from build123d import *

# Parameters (mm, degrees)
F0_R     = 30
F1_DEPTH = 1
F2_R     = 22.5
F3_DEPTH = 24
F5_R     = 20
F6_DEPTH = 25.001


# Not quite as in the source:
# - the program builds the solid bodies; features that only make, move or delete a surface that nothing else refers to are left out


with BuildPart() as f1:
    # F0 (on Front) → F1 (new body)
    with BuildSketch(Plane.XZ):
        Circle(F0_R)
    extrude(amount=F1_DEPTH)

    # F2 (on face) → F3 (join)
    with BuildSketch(Plane.XZ.offset(1)):
        Circle(F2_R)
    extrude(amount=F3_DEPTH)

    # F5 (on face) → F6 (cut, through all)
    with BuildSketch(Plane.XZ.offset(25)):
        Circle(F5_R)
    extrude(amount=-F6_DEPTH, mode=Mode.SUBTRACT)


solid = f1.part
Work out the finished part from the listing and answer in its coordinate system (mm). A direction names the side the tool comes from. Coordinates: 2 decimals unless noted, no trailing zeros. Write each loop counter-clockwise with the first axis right and the second up, starting at its lowest first coordinate (ties: lowest second). Pieces come first, ordered by that corner, then holes. Notation, with made-up numbers: M 35,34 L 57,34 A19 ccw 57,70 Z; hole C 47.25,81.5 d10. An arc over 180 degrees is marked long. Write item = value, one per line.
1. Straight lines are drawn through the part: line 1 (Z direction, x = 0, y = -15.75); line 2 (Z direction, x = 9, y = -17.25); line 3 (Y direction, x = 24.5, z = 1). For each, find the intervals that lie inside material, in ascending order. Write a range as from..to.
Solution:
line_1 = -22.5..-20, 20..22.5
line_2 = -20.62..-17.86, 17.86..20.62
line_3 = -1..0
2. The part is cut by section A-A (z = 0). Determine the outline of the cut face in (x, y), then the cut area to 3 significant figures.
Solution:
outline = M -30,-1 L -22.5,-1 L -22.5,-25 L -20,-25 L -20,0 L -30,0 Z; M 20,-25 L 22.5,-25 L 22.5,-1 L 30,-1 L 30,0 L 20,0 Z
area = 140 mm2
3. The part is cut by section D-D (x = -21.5). Determine the outline of the cut face in (y, z), then the cut area to 3 significant figures.
Solution:
outline = M -25,-6.63 L -1,-6.63 L -1,-20.92 L 0,-20.92 L 0,20.92 L -1,20.92 L -1,6.63 L -25,6.63 Z
area = 360 mm2
4. For faces 4 (the face through (6, 0, -20)), 5 (the face through (10.382, -12.832, -19.961)), determine the directions among +Z, -Z, +X, -X, +Y, -Y from which every point of the face is accessible in a straight line to the end or side of a thin tool.
Solution:
face_4 = +Z, -Z, +X, -X, +Y
face_5 = -Y
5. The part is cut by section B-B (x = 0). Determine the outline of the cut face in (y, z), then the cut area to 3 significant figures.
Solution:
outline = M -25,-22.5 L -1,-22.5 L -1,-30 L 0,-30 L 0,-20 L -25,-20 Z; M -25,20 L 0,20 L 0,30 L -1,30 L -1,22.5 L -25,22.5 Z
area = 140 mm2
6. The part is cut by section C-C (y = -20.75). Determine the outline of the cut face in (x, z), then the cut area to 3 significant figures.
Solution:
outline = C 0,0 d45; hole C 0,0 d40
area = 334 mm2
7. Determine the mould class of faces 1 (the face through (-4.336, -12.675, -19.524)), 2 (the face through (4.3, -1, 22.4)), 3 (the face through (-29.97, -0.49, 1.32)) for opening direction X: released by +X, released by -X, zero draft, split by the parting line, or undercut.
Solution:
face_1 = undercut
face_2 = zero draft
face_3 = split by the parting line
8. Flat-ended cylindrical pins translate along their axes: pin 1 (1 mm diameter, centred on x = 6.5, y = -22.5, fed in from +Z); pin 2 (8 mm diameter, centred on y = -10, z = -0.5, fed in from +X); pin 3 (1.5 mm diameter, centred on x = -20, y = -8.5, fed in from -Z); pin 4 (24 mm diameter, centred on x = 0, z = 0, fed in from -Y). Find the tip coordinate at first contact, or state that the pin passes through.
Solution:
pin_1 = 21.69
pin_2 = 22.5
pin_3 = -11.65
pin_4 = through
